Could you check a few things on this model? Use its own coordinates, in mm. A direction names the side the tool comes from. Round coordinates to 2 decimals unless told otherwise and drop trailing zeros. Loops run counter-clockwise (first coordinate to the right, second up) from the corner with the lowest first, then second, coordinate; pieces in that order, holes last. Notation, with made-up numbers: (-29.5, -23.75) -> (23.5, -23.75) arc R22 ccw to (23.5, -8.75) -> close; hole circle Ø6 at (45.5, 42.5). An arc over 180 degrees is marked (long way). Put each result on its own line as item: value. Start each with the question number.
1. Imagine slicing it at C-C, the plane x = 30. Please give me the cut outline in (y, z).
2. Imagine slicing it at D-D, the plane z = -27. Please give me the cut outline in (x, y).
3. Imagine slicing it at B-B, the plane y = 1.25. Count the separate pieces of the cut face and the enclosed holes in it, and give its area (3 significant figures).
4. Which directions (+Z, -Z, +X, -X, +Y, -Y) give clear straight access to the entire face, cutting with the end or side of a thin tool? Please do faces 1 (the flat face through (-7, 0, 0)), 2 (the cylindrical face through (0, 7.5, -2.5)), 3 (the flat face through (0, 8, -1.5)).
5. I'm going to push flat-ended pins straight in: P1, Ø0.9, axis at x = 0.5, y = 4, coming from the +Z side; P2, Ø5, axis at x = -6, y = 2, coming from the -Z side; P3, Ø3.5, axis at x = 30, z = 0, coming from the +Y side. Where does each tip first touch, or does it pass through?
6. I need wall thicknesses on line 1 (Y direction, x = -19.5, z = -0.5); line 2 (Z direction, x = 10, y = 1.65); line 3 (Z direction, x = 0, y = 5.8). Which ranges of each line are inside material? Lowest first, please. Write a range as [from, to].
7. If we mould it in two halves opening along Y, with no side actions, what happens to faces 4 (the cylindrical face through (0, 4.5, -2.5)), 5 (the flat face through (-7, 3, 0)), 6 (the flat face through (0, 2, -1.5))? For each: pulls with the +Y half, pulls with the -Y half, needs draft (parallel to the pull), parting line crosses it, or undercut.
8. Imagine slicing it at A-A, the plane x = 10. Please give me the cut outline in (y, z), and give its area (3 significant figures).
```python
from build123d import *
from build123d.topology import SkipClean

# Parameters (mm, degrees)
SKETCH_1_R          = 35
EXTRUDE_1_DEPTH     = 3
CUT_EXTRUDE_1_DEPTH = 3
EXTRUDE_START       = 6
EXTRUDE_2_DEPTH     = 6
CUT_EXTRUDE_START   = -2.0000001
CUT_EXTRUDE_2_DEPTH = 2.0000001
SKETCH_5_R          = 1.55
CUT_EXTRUDE_3_DEPTH = 6


# Read off the part's stored shape, not the designer's step: the extrude step
with BuildPart() as part:
    # Sketch 1 → Extrude 1 (new body)
    with BuildSketch(Plane(origin=(0, 0, 0), x_dir=(1, 0, 0), z_dir=(0, 1, 0))):
        with Locations(Location((0, 0, 0), (0, 0, 270))):
            Circle(SKETCH_1_R)
    extrude(amount=EXTRUDE_1_DEPTH)

    # Sketch 2 → Cut-Extrude 1 (cut)
    with BuildSketch(Plane(origin=(0, 3, 0), x_dir=(1, 0, 0), z_dir=(0, 1, 0))):
        with BuildLine():
            Line((0, 1.5), (-1.469693846, 1.5))
            ThreePointArc((-1.469693846, 1.5), (-0.8135241, -1.936021317), (2.1, 0))
            ThreePointArc((2.1, 0), (1.936021317, 0.8135241), (1.469693846, 1.5))
            Line((1.469693846, 1.5), (0, 1.5))
        make_face()
    extrude(amount=-CUT_EXTRUDE_1_DEPTH, mode=Mode.SUBTRACT)

    # Sketch 3 → Extrude 2 (add)
    with BuildSketch(Plane(origin=(0, 3, 0), x_dir=(1, 0, 0), z_dir=(0, 1, 0)).offset(EXTRUDE_START)):
        with BuildLine():
            Line((-1.469693846, 1.5), (-3.16227766, 1.5))
            ThreePointArc((-3.16227766, 1.5), (-0.768774411, -3.414525722), (3.5, 0))
            ThreePointArc((3.5, 0), (3.414525722, 0.768774411), (3.16227766, 1.5))
            Line((3.16227766, 1.5), (1.469693846, 1.5))
            ThreePointArc((1.469693846, 1.5), (0, -2.1), (-1.469693846, 1.5))
        make_face()
        with BuildLine():
            ThreePointArc((3.16227766, 1.5), (0, 3.5), (-3.16227766, 1.5))
            Line((-3.16227766, 1.5), (-1.469693846, 1.5))
            Line((-1.469693846, 1.5), (-1.322875656, 1.5))
            ThreePointArc((-1.322875656, 1.5), (0, 2), (1.322875656, 1.5))
            Line((1.322875656, 1.5), (1.469693846, 1.5))
            Line((1.469693846, 1.5), (3.16227766, 1.5))
        make_face()
        with BuildLine():
            ThreePointArc((1.322875656, 1.5), (0, 2), (-1.322875656, 1.5))
            Line((-1.322875656, 1.5), (0, 1.5))
            Line((0, 1.5), (1.322875656, 1.5))
        make_face()
    extrude(amount=-EXTRUDE_2_DEPTH)

    # Cut-Extrude 2 outline → Cut-Extrude 2 (cut)
    with BuildSketch(Plane.XY.offset(-1.5).offset(CUT_EXTRUDE_START)):
        with BuildLine():
            ThreePointArc((-1.469693846, 5.7), (0, 4.5), (1.469693846, 5.7))
            Line((1.469693846, 5.7), (1.469693846, 6.3))
            ThreePointArc((1.469693846, 6.3), (0, 7.5), (-1.469693846, 6.3))
            Line((-1.469693846, 6.3), (-1.469693846, 5.7))
        make_face()
    extrude(amount=CUT_EXTRUDE_2_DEPTH, mode=Mode.SUBTRACT)

    # Sketch 5 → Cut-Extrude 3 (cut)
    with SkipClean():  # the faces are left unmerged after this step: merging them gives an invalid solid
        with BuildSketch(Plane(origin=(0, 3, 0), x_dir=(1, 0, 0), z_dir=(0, 1, 0))):
            with BuildLine():
                ThreePointArc((1.55, -30), (1.096015511, -28.903984489), (0, -28.45))
                Line((0, -28.45), (0, -31.55))
                ThreePointArc((0, -31.55), (1.096015511, -31.096015511), (1.55, -30))
            make_face()
            with BuildLine():
                Line((0, -31.55), (0, -28.45))
                ThreePointArc((0, -28.45), (-1.55, -30), (0, -31.55))
            make_face()
            with BuildLine():
                ThreePointArc((1.55, -10), (1.096015511, -8.903984489), (0, -8.45))
                Line((0, -8.45), (0, -11.55))
                ThreePointArc((0, -11.55), (1.096015511, -11.096015511), (1.55, -10))
            make_face()
            with BuildLine():
                Line((0, -11.55), (0, -8.45))
                ThreePointArc((0, -8.45), (-1.55, -10), (0, -11.55))
            make_face()
            with Locations(Location((21.213203436, -21.213203436, 0), (0, 0, 270))):
                Circle(SKETCH_5_R)
            with BuildLine():
                ThreePointArc((31.55, 0), (30, 1.55), (28.45, 0))
                Line((28.45, 0), (31.55, 0))
            make_face()
            with BuildLine():
                Line((31.55, 0), (28.45, 0))
                ThreePointArc((28.45, 0), (30, -1.55), (31.55, 0))
            make_face()
            with Locations(Location((21.213203436, 21.213203436, 0), (0, 0, 270))):
                Circle(SKETCH_5_R)
            with BuildLine():
                ThreePointArc((0, 31.55), (-1.55, 30), (0, 28.45))
                Line((0, 28.45), (0, 30))
                Line((0, 30), (0, 31.55))
            make_face()
            with BuildLine():
                Line((0, 30), (0, 28.45))
                ThreePointArc((0, 28.45), (1.096015511, 28.903984489), (1.55, 30))
                ThreePointArc((1.55, 30), (1.096015511, 31.096015511), (0, 31.55))
                Line((0, 31.55), (0, 30))
            make_face()
            with BuildLine():
                ThreePointArc((11.55, 0), (10, 1.55), (8.45, 0))
                Line((8.45, 0), (11.55, 0))
            make_face()
            with BuildLine():
                Line((11.55, 0), (8.45, 0))
                ThreePointArc((8.45, 0), (10, -1.55), (11.55, 0))
            make_face()
            with BuildLine():
                ThreePointArc((0, 11.55), (-1.55, 10), (0, 8.45))
                Line((0, 8.45), (0, 10))
                Line((0, 10), (0, 11.55))
            make_face()
            with BuildLine():
                Line((0, 10), (0, 8.45))
                ThreePointArc((0, 8.45), (1.096015511, 8.903984489), (1.55, 10))
                ThreePointArc((1.55, 10), (1.096015511, 11.096015511), (0, 11.55))
                Line((0, 11.55), (0, 10))
            make_face()
            with Locations(Location((-21.213203436, -21.213203436, 0), (0, 0, 270))):
                Circle(SKETCH_5_R)
            with Locations(Location((-21.213203436, 21.213203436, 0), (0, 0, 270))):
                Circle(SKETCH_5_R)
            with BuildLine():
                ThreePointArc((-11.55, 0), (-10, -1.55), (-8.45, 0))
                Line((-8.45, 0), (-11.55, 0))
            make_face()
            with BuildLine():
                Line((-11.55, 0), (-8.45, 0))
                ThreePointArc((-8.45, 0), (-10, 1.55), (-11.55, 0))
            make_face()
            with BuildLine():
                ThreePointArc((-31.55, 0), (-30, -1.55), (-28.45, 0))
                Line((-28.45, 0), (-31.55, 0))
            make_face()
            with BuildLine():
                Line((-31.55, 0), (-28.45, 0))
                ThreePointArc((-28.45, 0), (-30, 1.55), (-31.55, 0))
            make_face()
        extrude(amount=-CUT_EXTRUDE_3_DEPTH, mode=Mode.SUBTRACT)


solid = part.part
```
Entries:
1. outline: (0, -18.03) -> (3, -18.03) -> (3, -1.55) -> (0, -1.55) -> close; (0, 1.55) -> (3, 1.55) -> (3, 18.03) -> (0, 18.03) -> close
2. outline: (-22.27, 0) -> (22.27, 0) -> (22.27, 3) -> (-22.27, 3) -> close
3. separate pieces: 1
3. enclosed holes: 13
3. area: 3,750 mm^2
4. face 1: +Z, -Z, +X, -X, -Y
4. face 2: -Z
4. face 3: +Y, -Y
5. P1: z = 3.5
5. P2: z = -34.82
5. P3: y = 3
6. line 1: [0, 3]
6. line 2: [-33.54, -1.55], [1.55, 33.54]
6. line 3: [2.1, 3.5]
7. face 4: undercut
7. face 5: pulls with the +Y half
7. face 6: needs draft
8. outline: (0, -33.54) -> (3, -33.54) -> (3, -1.55) -> (0, -1.55) -> close; (0, 1.55) -> (3, 1.55) -> (3, 33.54) -> (0, 33.54) -> close
8. area: 192 mm^2
